Geometry: final body of the model. Coordinates: model frame, mm. A direction names the side the tool comes from. Give positions to 0.01 mm unless a question says otherwise; leave off trailing zeros. Write each loop counter-clockwise with the first axis right and the second up, starting at its lowest first coordinate (ties: lowest second). Pieces come first, ordered by that corner, then holes. Notation, with made-up numbers: (74.25, 10.25) -> (117.25, 10.25) arc R17 cw to (117.25, 39.25) -> close; hole circle Ø5 at (-14, -37). An arc over 180 degrees is marked (long way). Answer as a JSON object with one key per item and string values.
Autodesk Inventor part; units mm, degrees
ref_plane "YZ Plane" through (0, 0, 0) normal (1, 0, 0) x (0, 1, 0)
ref_plane "XZ Plane" through (0, 0, 0) normal (0, 1, 0) x (-1, 0, 0)
ref_plane "XY Plane" through (0, 0, 0) normal (0, 0, 1) x (1, 0, 0)
sketch "Sketch2" plane through (0, 0, 0) normal (0, 0, 1) x (1, 0, 0)
  line L0 (0, 0) -> (-1022.35, 0)
  line L1 (-1022.35, 0) -> (-1022.35, 50.8)
  line L2 (-1022.35, 50.8) -> (0, 50.8)
  line L3 (0, 50.8) -> (0, 0)
  dimension "d0" = 50.8
  dimension "d1" = 1022.35
extrude "Extrusion1" add sketch "Sketch2" along normal blind 3.175
sketch "Sketch3" plane through (0, 0, 3.175) normal (0, 0, 1) x (1, 0, 0)
  line L0 (0, 50.8) -> (-1022.35, 50.8)
  line L1 (0, 0) -> (-3.175, 0)
  line L2 (-3.175, 0) -> (-3.175, 50.8)
  line L3 (-3.175, 50.8) -> (0, 50.8)
  line L4 (0, 50.8) -> (0, 0)
  line L5 (-1022.35, 50.8) -> (-1019.175, 50.8)
  line L6 (-1019.175, 50.8) -> (-1019.175, 0)
  line L7 (-1019.175, 0) -> (-1022.35, 0)
  line L8 (-1022.35, 0) -> (-1022.35, 50.8)
  dimension "d4" = 3.175
  dimension "d5" = 3.175
extrude "Extrusion2" add sketch "Sketch3" along normal blind 25.4
sketch "Sketch4" plane through (0, 0, 3.175) normal (0, 0, 1) x (1, 0, 0)
  line L0 (-1019.175, 0) -> (-1019.175, 50.8)
  line L1 (-1019.175, 50.8) -> (-1019.175, 0)
  line L2 (-3.175, 0) -> (-3.175, 50.8)
  circle A0 centre (-892.175, 25.4) radius 6.2992
  circle A1 centre (-130.175, 25.4) radius 6.2992
  line L3 (-1019.175, 0) -> (-3.175, 0)
  line L4 (-1019.175, 0) -> (-3.175, 0)
  point P0 (0, 0)
  dimension "d8" = 12.5984
  dimension "d9" = 12.5984
  dimension "d10" = 25.4
  dimension "d11" = 127
  dimension "d12" = 127
  dimension "d13" = 25.4
properties part number "Bumpers"
Q1. Cut plane C-C (x = -305). Return the cut outline in (y, z) (3 decimals), and give its area (3 significant figures).
Values:
{"outline": "(0, 0) -> (50.8, 0) -> (50.8, 3.175) -> (0, 3.175) -> close", "area": "161 mm²"}
Q2. Material intervals for L1, parallel to X at y = 3.5, z = 5.25 (3 decimals); L2, parallel to Z at x = -413, y = 27 (3 decimals), sorted ascending. Write a range as from..to.
Values:
{"L1": "-1022.35..-1019.175, -3.175..0", "L2": "0..3.175"}
Q3. Cut plane B-B (y = 29.5). Return the cut outline in (x, z) (3 decimals).
Values:
{"outline": "(-1022.35, 0) -> (0, 0) -> (0, 28.575) -> (-3.175, 28.575) -> (-3.175, 3.175) -> (-1019.175, 3.175) -> (-1019.175, 28.575) -> (-1022.35, 28.575) -> close"}
Q4. Cut plane A-A (z = 10). Return the cut outline in (x, y) (3 decimals).
Values:
{"outline": "(-1022.35, 0) -> (-1019.175, 0) -> (-1019.175, 50.8) -> (-1022.35, 50.8) -> close; (-3.175, 0) -> (0, 0) -> (0, 50.8) -> (-3.175, 50.8) -> close"}
Q5. First-contact query: P1, Ø5, axis at y = 18, z = 10, coming from the +X side; P2, Ø3, axis at x = -552.5, y = 20.5, coming from the +Z side (3 decimals). Flat tips, straight axial feed; report the tip coordinate or a pass-through.
Values:
{"P1": "x = 0", "P2": "z = 3.175"}
Q6. Set-up query: faces 5 (the flat face through (-509, 0, 2)), 6 (the flat face through (-518, 26, 3.175)). Return all of +Z, -Z, +X, -X, +Y, -Y with unobstructed straight access to the full face (end or side cutting, diameter ignored); none if empty.
Values:
{"face 5": "+Z, -Z, +X, -X, -Y", "face 6": "+Z, +Y, -Y"}
Q7. Mould query, pull axis X, two halves, no side actions, for faces 1 (the flat face through (-1019.175, 26, 16)), 2 (the flat face through (-3.175, 25, 16)), 3 (the flat face through (-1022.35, 25, 14)), 4 (the flat face through (-518, 26, 0)). Classes: pulls with the +X half, pulls with the -X half, needs draft (parallel to the pull), parting line crosses it, or undercut.
Values:
{"face 1": "undercut", "face 2": "undercut", "face 3": "pulls with the -X half", "face 4": "needs draft"}
